```python
from build123d import *

# Parameters (mm, degrees)
RESSALTO_EXTRUS_O2_DEPTH      = 30
RESSALTO_EXTRUS_O3_START      = 3
RESSALTO_EXTRUS_O3_DEPTH      = 3
RESSALTO_EXTRUS_O4_DEPTH      = 3
RESSALTO_EXTRUS_O4_DEPTH_BACK = 10
CORTE_EXTRUS_O1_DEPTH         = 10
CORTE_EXTRUS_O2_REACH         = 83.702
FILETE1_START                 = -19.773073923
FILETE1_DEPTH                 = 36.75
FILETE1_START_2               = -13.40159992
FILETE1_2_DEPTH               = 59


with BuildPart() as part:
    # Esboço2 → Ressalto-extrusão2 (new body)
    with BuildSketch(Plane(origin=(0, 0, 0), x_dir=(0, 0, -1), z_dir=(1, 0, 0))):
        with BuildLine():
            Line((2.90159992, -0.062465938), (-35.09840008, -0.062465938))
            Line((-35.09840008, -0.062465938), (-39.886084903, -0.062465938))
            ThreePointArc((-39.886084903, -0.062465938), (-45.202180234, 1.467638524), (-48.891439328, 5.589707975))
            ThreePointArc((-48.891439328, 5.589707975), (-52.096536948, 9.772081499), (-56.69840008, 12.338743681))
            ThreePointArc((-56.69840008, 12.338743681), (-59.373224015, 11.895603401), (-60.59840008, 9.476926077))
            Line((-60.59840008, 9.476926077), (-60.59840008, 20.976926077))
            ThreePointArc((-60.59840008, 20.976926077), (-59.719720424, 23.09824642), (-57.59840008, 23.976926077))
            Line((-57.59840008, 23.976926077), (25.40159992, 23.976926077))
            ThreePointArc((25.40159992, 23.976926077), (27.522920263, 23.09824642), (28.40159992, 20.976926077))
            Line((28.40159992, 20.976926077), (28.40159992, 9.476926077))
            ThreePointArc((28.40159992, 9.476926077), (27.176423855, 11.895603401), (24.50159992, 12.338743681))
            ThreePointArc((24.50159992, 12.338743681), (19.899736788, 9.772081499), (16.694639168, 5.589707975))
            ThreePointArc((16.694639168, 5.589707975), (13.005380073, 1.467638524), (7.689284743, -0.062465938))
            Line((7.689284743, -0.062465938), (2.90159992, -0.062465938))
        make_face()
    extrude(amount=RESSALTO_EXTRUS_O2_DEPTH)

    # Esboço3 → Ressalto-extrusão3 (add)
    with BuildSketch(Plane.ZY.offset(RESSALTO_EXTRUS_O3_START)):
        with BuildLine():
            Line((60.59840008, 15.226926077), (60.59840008, 20.976926077))
            ThreePointArc((60.59840008, 20.976926077), (59.719720424, 23.09824642), (57.59840008, 23.976926077))
            Line((57.59840008, 23.976926077), (16.09840008, 23.976926077))
            Line((16.09840008, 23.976926077), (-25.40159992, 23.976926077))
            ThreePointArc((-25.40159992, 23.976926077), (-27.522920263, 23.09824642), (-28.40159992, 20.976926077))
            Line((-28.40159992, 20.976926077), (-28.40159992, 15.226926077))
            Line((-28.40159992, 15.226926077), (-28.40159992, -16.773073923))
            ThreePointArc((-28.40159992, -16.773073923), (-27.522920263, -18.894394267), (-25.40159992, -19.773073923))
            Line((-25.40159992, -19.773073923), (57.59840008, -19.773073923))
            ThreePointArc((57.59840008, -19.773073923), (59.719720424, -18.894394267), (60.59840008, -16.773073923))
            Line((60.59840008, -16.773073923), (60.59840008, 15.226926077))
        make_face()
    extrude(amount=-RESSALTO_EXTRUS_O3_DEPTH)

    # Esboço4 → Ressalto-extrusão4 (add, two sides: drawn at the far end of the back side and taken through both)
    with BuildSketch(Plane(origin=(30, 0, 0), x_dir=(0, 0, -1), z_dir=(1, 0, 0)).offset(-RESSALTO_EXTRUS_O4_DEPTH_BACK)):
        with BuildLine():
            Line((-16.09840008, 23.976926077), (25.40159992, 23.976926077))
            ThreePointArc((25.40159992, 23.976926077), (27.522920263, 23.09824642), (28.40159992, 20.976926077))
            Line((28.40159992, 20.976926077), (28.40159992, 15.226926077))
            Line((28.40159992, 15.226926077), (28.40159992, -16.773073923))
            ThreePointArc((28.40159992, -16.773073923), (27.522920263, -18.894394267), (25.40159992, -19.773073923))
            Line((25.40159992, -19.773073923), (-57.59840008, -19.773073923))
            ThreePointArc((-57.59840008, -19.773073923), (-59.719720424, -18.894394267), (-60.59840008, -16.773073923))
            Line((-60.59840008, -16.773073923), (-60.59840008, 15.226926077))
            Line((-60.59840008, 15.226926077), (-60.59840008, 20.976926077))
            ThreePointArc((-60.59840008, 20.976926077), (-59.719720424, 23.09824642), (-57.59840008, 23.976926077))
            Line((-57.59840008, 23.976926077), (-16.09840008, 23.976926077))
        make_face()
    extrude(amount=RESSALTO_EXTRUS_O4_DEPTH + RESSALTO_EXTRUS_O4_DEPTH_BACK)

    # Esboço8 → Corte-extrusão1 (cut)
    with BuildSketch(Plane(origin=(33, 0, 0), x_dir=(0, 0, -1), z_dir=(1, 0, 0))):
        with BuildLine():
            Line((-43.59840008, -2.773073923), (11.40159992, -2.773073923))
            ThreePointArc((11.40159992, -2.773073923), (12.815813482, -3.358860361), (13.40159992, -4.773073923))
            Line((13.40159992, -4.773073923), (13.40159992, -10.773073923))
            ThreePointArc((13.40159992, -10.773073923), (12.815813482, -12.187287486), (11.40159992, -12.773073923))
            Line((11.40159992, -12.773073923), (-43.59840008, -12.773073923))
            ThreePointArc((-43.59840008, -12.773073923), (-45.012613643, -12.187287486), (-45.59840008, -10.773073923))
            Line((-45.59840008, -10.773073923), (-45.59840008, -4.773073923))
            ThreePointArc((-45.59840008, -4.773073923), (-45.012613643, -3.358860361), (-43.59840008, -2.773073923))
        make_face()
        with BuildLine():
            Line((-43.59840008, 6.976926077), (11.40159992, 6.976926077))
            ThreePointArc((11.40159992, 6.976926077), (12.815813482, 7.562712514), (13.40159992, 8.976926077))
            Line((13.40159992, 8.976926077), (13.40159992, 14.976926077))
            ThreePointArc((13.40159992, 14.976926077), (12.815813482, 16.391139639), (11.40159992, 16.976926077))
            Line((11.40159992, 16.976926077), (-43.59840008, 16.976926077))
            ThreePointArc((-43.59840008, 16.976926077), (-45.012613643, 16.391139639), (-45.59840008, 14.976926077))
            Line((-45.59840008, 14.976926077), (-45.59840008, 8.976926077))
            ThreePointArc((-45.59840008, 8.976926077), (-45.012613643, 7.562712514), (-43.59840008, 6.976926077))
        make_face()
    extrude(amount=-CORTE_EXTRUS_O1_DEPTH, mode=Mode.SUBTRACT)

    # Corte-extrusão2: up to this face of the body (flat: up to its plane)
    corte_extrus_o2_end = Plane(part.part.faces().sort_by_distance((28, 16.976926077, 16.09840008))[0])
    # Esboço9 → Corte-extrusão2 (cut, up to the picked face)
    with BuildSketch(Plane(origin=(0, -19.773073923, 0), x_dir=(-1, 0, 0), z_dir=(0, -1, 0)), mode=Mode.PRIVATE) as corte_extrus_o2_sk1:
        with BuildLine():
            Line((-25, 13.40159992), (-28, 13.40159992))
            ThreePointArc((-28, 13.40159992), (-29.414213562, 12.815813482), (-30, 11.40159992))
            Line((-30, 11.40159992), (-30, -43.59840008))
            ThreePointArc((-30, -43.59840008), (-29.414213562, -45.012613643), (-28, -45.59840008))
            Line((-28, -45.59840008), (-25, -45.59840008))
            ThreePointArc((-25, -45.59840008), (-23.585786438, -45.012613643), (-23, -43.59840008))
            Line((-23, -43.59840008), (-23, 11.40159992))
            ThreePointArc((-23, 11.40159992), (-23.585786438, 12.815813482), (-25, 13.40159992))
        make_face()
    corte_extrus_o2_tool1 = split(extrude(corte_extrus_o2_sk1.sketch, amount=-CORTE_EXTRUS_O2_REACH, mode=Mode.PRIVATE), bisect_by=corte_extrus_o2_end, keep=Keep.BOTH, mode=Mode.PRIVATE)
    add(corte_extrus_o2_tool1.solids().sort_by(Axis((26.5, -19.773074, 16.0984), (0, 1, 0)))[0], mode=Mode.SUBTRACT)

    # Filete1: read off the stored shape, not the designer's step
    # Filete1 outline → Filete1 (add)
    with BuildSketch(Plane(origin=(0, 0, 0), x_dir=(1, 0, 0), z_dir=(0, 1, 0)).offset(FILETE1_START)):
        with BuildLine():
            ThreePointArc((25, -45.59840008), (23.585786437, -45.012613642), (23, -43.59840008))
            Line((23, -43.59840008), (23, -45.59840008))
            Line((23, -45.59840008), (25, -45.59840008))
        make_face()
        with BuildLine():
            ThreePointArc((23, 11.40159992), (23.585786438, 12.815813482), (25, 13.40159992))
            Line((25, 13.40159992), (23, 13.40159992))
            Line((23, 13.40159992), (23, 11.40159992))
        make_face()
    extrude(amount=FILETE1_DEPTH)

    # Filete1 2 outline → Filete1 2 (add)
    with BuildSketch(Plane.XY.offset(FILETE1_START_2)):
        with BuildLine():
            ThreePointArc((23, 14.976926077), (23.585786438, 16.391139639), (25, 16.976926077))
            Line((25, 16.976926077), (23, 16.976926077))
            Line((23, 16.976926077), (23, 14.976926077))
        make_face()
    extrude(amount=FILETE1_2_DEPTH)


solid = part.part
```
Check sheet for the modelled part. Datum: model origin and axes. Units: mm. A direction names the side the tool comes from. Round coordinates to 2 decimals unless told otherwise and drop trailing zeros. Write each loop counter-clockwise with the first axis right and the second up, starting at its lowest first coordinate (ties: lowest second). Pieces come first, ordered by that corner, then holes. Notation, with made-up numbers: M 70,28 L 127,28 A23 ccw 127,67 Z; hole C 8,53 d11. An arc over 180 degrees is marked long. Write item = value, one per line. Start each with the question number.
1. Section check C-C, the plane x = 10. Record the cut outline in (y, z), then the cut area to 3 significant figures.
2. Tool access check on faces 4 (the cylindrical face through (31.091, -3.374, 45.028)), 5 (the cylindrical face through (9.86, 1.43, 45.14)), 6 (the flat face through (27, -1, -13.402)), 7 (the cylindrical face through (29.4, 2.01, -12.83)). Record the directions out of +Z, -Z, +X, -X, +Y, -Y that give a thin tool (end or side, any length) a straight path to the whole face; none if there is none.
3. Section check A-A, the plane y = -1. Record the cut outline in (x, z), then the cut area to 3 significant figures.
4. Scan lines: line 1 (Y direction, x = 30.5, z = 21); line 2 (X direction, y = -15.5, z = 32.5); line 3 (X direction, y = -9.5, z = -20). Record each from-to range of solid material in increasing order. Write a range as [from, to].
5. Gauge pin test, flat ends, axial feed: pin 1 (12 mm diameter, centred on x = 18, y = -15, fed in from -Z); pin 2 (1 mm diameter, centred on x = 18.5, y = -7.5, fed in from +Z). Record the tip position at first contact, or that the pin passes through.
6. Section check D-D, the plane y = 13.5. Record the cut outline in (x, z), then the cut area to 3 significant figures.
7. Section check B-B, the plane z = 7. Record the cut outline in (x, y).
8. Release check for a two-part mould opening along X. For faces 1 (the cylindrical face through (31.1, -12.2, 45)), 2 (the flat face through (-3, 2, 15)), 3 (the flat face through (30, 2, 16)) record: pulls with the +X half, pulls with the -X half, needs draft (parallel to the pull), parting line crosses it, or undercut.
Results found:
q1.outline = M -0.06,-7.69 A10 ccw 5.59,-16.69 A13 cw 12.34,-24.5 A3 cw 9.48,-28.4 L 20.98,-28.4 A3 ccw 23.98,-25.4 L 23.98,57.6 A3 ccw 20.98,60.6 L 9.48,60.6 A3 cw 12.34,56.7 A13 cw 5.59,48.89 A10 ccw -0.06,39.89 Z
q1.area = 1,860 mm^2
q2.face_4 = +X
q2.face_5 = +Z, -Y
q2.face_6 = none
q2.face_7 = -Y
q3.outline = M -3,-28.4 L 0,-28.4 L 0,60.6 L -3,60.6 Z; M 20,-28.4 L 33,-28.4 L 33,60.6 L 20,60.6 Z; hole M 23,-11.4 A2 ccw 25,-13.4 L 28,-13.4 A2 ccw 30,-11.4 L 30,43.6 A2 ccw 28,45.6 L 25,45.6 A2 ccw 23,43.6 Z
q3.area = 1,010 mm^2
q4.line_1 = [-19.77, -12.77], [-2.77, 6.98], [16.98, 23.98]
q4.line_2 = [-3, 0], [20, 23], [30, 33]
q4.line_3 = [-3, 0], [20, 33]
q5.pin_1 = -28.4
q5.pin_2 = through
q6.outline = M -3,-28.4 L 33,-28.4 L 33,-13.4 L 25,-13.4 A2 cw 23,-11.4 L 23,43.6 A2 cw 25,45.6 L 33,45.6 L 33,60.6 L -3,60.6 Z
q6.area = 2,620 mm^2
q7.outline = M -3,-19.77 L 0,-19.77 L 0,-0.06 L 20,-0.06 L 20,-19.77 L 23,-19.77 L 23,14.98 A2 cw 25,16.98 L 33,16.98 L 33,23.98 L -3,23.98 Z; M 30,-19.77 L 33,-19.77 L 33,-12.77 L 30,-12.77 Z; M 30,-2.77 L 33,-2.77 L 33,6.98 L 30,6.98 Z
q8.face_1 = needs draft
q8.face_2 = pulls with the -X half
q8.face_3 = undercut
